Read the model definition and answer for the solid it produces. Units are mm, in the model's axes. Give positions to 0.01 mm unless a question says otherwise; leave off trailing zeros. Order: outer loops, then holes, each group sorted by start corner. A loop starts at its lowest first (then second) coordinate and runs counter-clockwise, first axis right, second up. Notation, with made-up numbers: (37, 51.25) - (70, 51.25) arc R16 ccw to (70, 59.25) - close; hole circle Ø4 at (44, 39.25). An arc over 180 degrees is marked (long way). Write each question's results on one line, items separated by ' | '. Start each with the question number.
Q1. Find section B-B on z = -20.5. Give the vertices of the cut face in (x, y).
Q2. Flat-ended cylindrical pins translate along their axes: P1, Ø3, axis at x = 86, z = -13.5, coming from the +Y side; P2, Ø1, axis at y = 1.5, z = 27, coming from the +X side. Find the tip coordinate at first contact, or state that the pin passes through.
Q3. Find section A-A on z = 11. Give the vertices of the cut face in (x, y).
Q4. Find the intervals of material crossed by line 1 along Y through (x, z) = (-48, -8); line 2 along X through (y, z) = (7.5, -13); line 3 along X through (y, z) = (0.75, -7.5), in increasing order. Write a range as from..to.
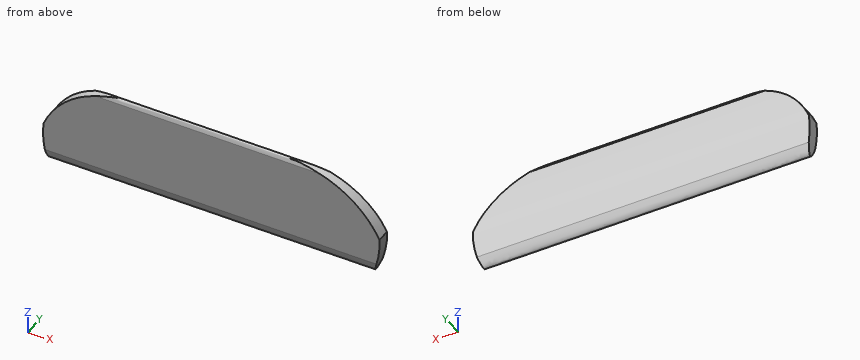
from build123d import *

# Parameters (mm, degrees)
SKETCH1_W                = 250
SKETCH1_H                = 70
BOSS_EXTRUDE1_DEPTH      = 10
CUT_EXTRUDE1_DEPTH       = 10
CUT_EXTRUDE2_DEPTH       = 10
CUT_EXTRUDE7_DEPTH       = 131.083540302
CUT_EXTRUDE7_DEPTH_BACK  = 131.083540302
CUT_EXTRUDE12_DEPTH      = 131.064564638
CUT_EXTRUDE12_DEPTH_BACK = 131.064564638
CUT_EXTRUDE15_DEPTH      = 10
CUT_EXTRUDE16_DEPTH      = 10
CUT_EXTRUDE21_DEPTH      = 131.064564638
CUT_EXTRUDE21_DEPTH_BACK = 131.064564638


with BuildPart() as part:
    # Sketch1 → Boss-Extrude1 (new body)
    with BuildSketch(Plane(origin=(0, 0, 0), x_dir=(1, 0, 0), z_dir=(0, 1, 0))):
        Rectangle(SKETCH1_W, SKETCH1_H)
    extrude(amount=BOSS_EXTRUDE1_DEPTH)

    # Sketch2 → Cut-Extrude1 (cut)
    with BuildSketch(Plane(origin=(0, 10, 0), x_dir=(1, 0, 0), z_dir=(0, 1, 0))):
        with BuildLine():
            Line((-125, -35), (-105.6811507, -35))
            ThreePointArc((-105.6811507, -35), (-123.319359291, -2.181448179), (-120.931126211, 35))
            Line((-120.931126211, 35), (-125, 35))
            Line((-125, 35), (-125, -35))
        make_face()
        with BuildLine():
            ThreePointArc((-102.585198357, -37.985491478), (-104.15687903, -36.517327288), (-105.6811507, -35))
            Line((-105.6811507, -35), (-125, -35))
            Line((-125, -35), (-125, 35))
            Line((-125, 35), (-120.931126211, 35))
            ThreePointArc((-120.931126211, 35), (-117.77369036, 42.419291873), (-113.756908851, 49.410769495))
            ThreePointArc((-113.756908851, 49.410769495), (-123.297106068, 68.789133967), (-141.939517672, 79.697702256))
            ThreePointArc((-141.939517672, 79.697702256), (-176.738011892, 49.445919486), (-154.950429467, 8.808414484))
            ThreePointArc((-154.950429467, 8.808414484), (-179.373061386, -41.265354418), (-129.299292485, -65.687986337))
            ThreePointArc((-129.299292485, -65.687986337), (-103.552743859, -63.784193915), (-102.585198357, -37.985491478))
        make_face()
    extrude(amount=-CUT_EXTRUDE1_DEPTH, mode=Mode.SUBTRACT)

    # Sketch3 → Cut-Extrude2 (cut)
    with BuildSketch(Plane(origin=(0, 10, 0), x_dir=(1, 0, 0), z_dir=(0, 1, 0))):
        with BuildLine():
            ThreePointArc((107.670924145, -35.29278609), (124.046120338, -1.80913671), (119.157389799, 35.142211572))
            ThreePointArc((119.157389799, 35.142211572), (134.08963077, 47.557806696), (153.427471124, 45.778269352))
            ThreePointArc((153.427471124, 45.778269352), (237.062768876, 49.332031087), (168.624576004, 1.127197211))
            ThreePointArc((168.624576004, 1.127197211), (150.729727191, -38.140394783), (107.670924145, -35.29278609))
        make_face()
    extrude(amount=-CUT_EXTRUDE2_DEPTH, mode=Mode.SUBTRACT)

    # Sketch7 → Cut-Extrude7 (cut, two sides: drawn at the far end of the back side and taken through both)
    with BuildSketch(Plane(origin=(0, 0, 0), x_dir=(0, 0, -1), z_dir=(1, 0, 0)).offset(-CUT_EXTRUDE7_DEPTH_BACK)):
        with BuildLine():
            ThreePointArc((33.533398698, 7.292236255), (-1.467141086, 9.688614292), (-36.298819038, 5.501177851))
            ThreePointArc((-36.298819038, 5.501177851), (-59.137780951, 12.031911856), (-75.102753404, 29.621349666))
            ThreePointArc((-75.102753404, 29.621349666), (-94.212515617, 81.478521501), (-38.963674899, 82.862314097))
            ThreePointArc((-38.963674899, 82.862314097), (26.341939645, 119.615559451), (63.095184998, 54.309944906))
            ThreePointArc((63.095184998, 54.309944906), (106.612811455, -5.853362128), (33.533398698, 7.292236255))
        make_face()
    extrude(amount=CUT_EXTRUDE7_DEPTH + CUT_EXTRUDE7_DEPTH_BACK, mode=Mode.SUBTRACT)

    # Sketch8 → Cut-Extrude12 (cut, two sides: drawn at the far end of the back side and taken through both)
    with BuildSketch(Plane(origin=(0, 0, 0), x_dir=(0, 0, -1), z_dir=(1, 0, 0)).offset(-CUT_EXTRUDE12_DEPTH_BACK)):
        with BuildLine():
            Line((-28.066580628, 7.960156192), (-42.709897039, 11.860300813))
            Line((-42.709897039, 11.860300813), (-42.709897039, -7.993078492))
            Line((-42.709897039, -7.993078492), (-28.71193991, -0.466643389))
            add(Edge.make_bspline(
                [(-28.066580628, 7.960156192), (-39.598055898, 0.513916796), (-33.220375755, 0.370849615), (-28.71193991, -0.466643389)],
                knots=[0, 0, 0, 0, 0.838507954, 0.838507954, 0.838507954, 0.838507954], degree=3))
        make_face()
    extrude(amount=CUT_EXTRUDE12_DEPTH + CUT_EXTRUDE12_DEPTH_BACK, mode=Mode.SUBTRACT)

    # Sketch9 → Cut-Extrude15 (cut)
    with BuildSketch(Plane(origin=(0, 0, 0), x_dir=(-1, 0, 0), z_dir=(0, -1, 0))):
        with BuildLine():
            Line((124.655946291, 5.484693498), (146.36395099, -21.002614193))
            Line((146.36395099, -21.002614193), (76.210821695, -48.228862541))
            Line((76.210821695, -48.228862541), (66.423803533, -43.378905656))
            Line((66.423803533, -43.378905656), (70.788178261, -34.57177278))
            ThreePointArc((70.788178261, -34.57177278), (103.40223816, -22.182216373), (124.655946291, 5.484693498))
        make_face()
    extrude(amount=-CUT_EXTRUDE15_DEPTH, mode=Mode.SUBTRACT)

    # Sketch10 → Cut-Extrude16 (cut)
    with BuildSketch(Plane(origin=(0, 0, 0), x_dir=(-1, 0, 0), z_dir=(0, -1, 0))):
        with BuildLine():
            Line((-57.675166137, -34.275423238), (-71.543821122, -47.200540174))
            Line((-71.543821122, -47.200540174), (-140.907758081, -43.326426614))
            Line((-140.907758081, -43.326426614), (-154.2664719, 14.83864241))
            Line((-154.2664719, 14.83864241), (-126.862900993, 9.383026654))
            ThreePointArc((-126.862900993, 9.383026654), (-98.892649646, -22.942974845), (-57.675166137, -34.275423238))
        make_face()
    extrude(amount=-CUT_EXTRUDE16_DEPTH, mode=Mode.SUBTRACT)

    # Sketch11 → Cut-Extrude21 (cut, two sides: drawn at the far end of the back side and taken through both)
    with BuildSketch(Plane(origin=(0, 0, 0), x_dir=(0, 0, -1), z_dir=(1, 0, 0)).offset(-CUT_EXTRUDE21_DEPTH_BACK)):
        with BuildLine():
            Line((25.230837074, 8.500137714), (41.025699478, 16.186384417))
            Line((41.025699478, 16.186384417), (42.557487911, 1.877911824))
            Line((42.557487911, 1.877911824), (37.210923704, -12.479147824))
            Line((37.210923704, -12.479147824), (27.144998545, -6.229370678))
            Line((27.144998545, -6.229370678), (24.539214353, -0.167468362))
            add(Edge.make_bspline(
                [(25.230837074, 8.500137714), (39.968005994, 2.152916652), (24.539214353, -0.167468362)],
                knots=[0, 0, 0, 1, 1, 1], degree=2))
        make_face()
    extrude(amount=CUT_EXTRUDE21_DEPTH + CUT_EXTRUDE21_DEPTH_BACK, mode=Mode.SUBTRACT)


solid = part.part
Working result:
1) outline: (-124.37, 0) - (123.77, 0) - (123.77, 8.96) - (-124.37, 8.96) - close
2) P1: y = 9.55 | P2: x = 92.59
3) outline: (-115.03, 0) - (113.35, 0) - (113.35, 9.2) - (-115.03, 9.2) - close
4) line 1: 0..9.69 | line 2: -124.87..124.73 | line 3: -124.71..124.88
